Geometry: see drawing. Coordinates: mm, zero at the bounding-box minimum. A direction names the side the tool comes from. Round coordinates to 2 decimals unless told otherwise and drop trailing zeros. Write each loop counter-clockwise with the first axis right and the second up, starting at its lowest first coordinate (ties: lowest second). Pieces come first, ordered by that corner, then holes. Notation, with made-up numbers: M 38,16.25 L 64,16.25 A32 ccw 64,55.25 Z; hole C 63,2 d7. An arc over 180 degrees is marked long. Use a Markdown table: item, result.
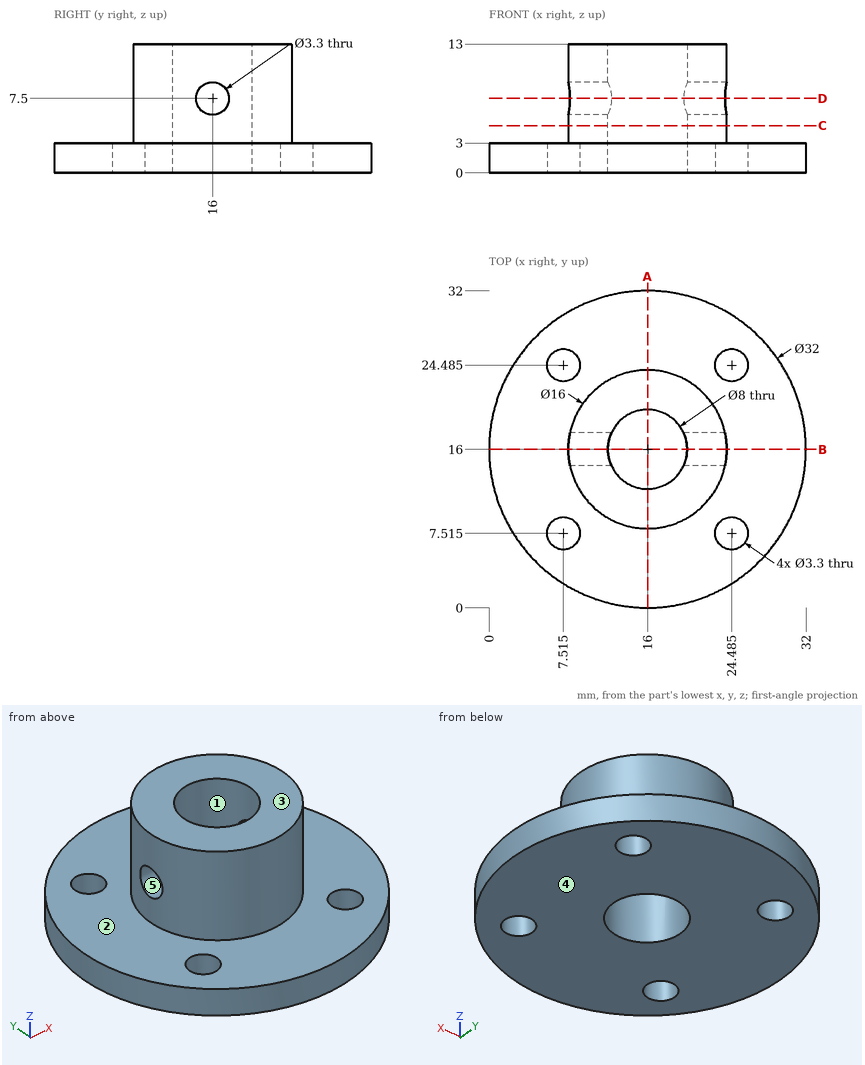
Q1. Mould query, pull axis Z, two halves, no side actions, for the marked faces 3, 4 and 5. Classes: +Z half, -Z half, draft (parallel to the pull), parting line (faces both ways), or undercut.
Results are:
| item | result |
|---|---|
| face 3 | +Z half |
| face 4 | -Z half |
| face 5 | undercut |
Q2. Section D-D on z = 7.5. Return loops of the section in (x, y), plus the area to 3 significant figures.
Results are:
| item | result |
|---|---|
| outline | M 8.17,14.35 A8 ccw 23.83,14.35 L 19.64,14.35 A4 cw 12.36,14.35 Z; M 8.17,17.65 L 12.36,17.65 A4 cw 19.64,17.65 L 23.83,17.65 A8 ccw Z |
| area | 124 mm^2 |
Q3. Section B-B on y = 16. Return loops of the section in (x, z), plus the area to 3 significant figures.
Results are:
| item | result |
|---|---|
| outline | M 0,0 L 12,0 L 12,5.85 L 8,5.85 L 8,3 L 0,3 Z; M 8,9.15 L 12,9.15 L 12,13 L 8,13 Z; M 20,0 L 32,0 L 32,3 L 24,3 L 24,5.85 L 20,5.85 Z; M 20,9.15 L 24,9.15 L 24,13 L 20,13 Z |
| area | 126 mm^2 |
Q4. First-contact query: pin 1 Ø5 at (x, y) = (9, 6.5) entering from +Z; pin 2 Ø4 at (y, z) = (16, 7.5) entering from -X; pin 3 Ø5 at (x, z) = (11.5, 9.5) entering from -Y. Flat tips, straight axial feed; report the tip coordinate or a pass-through.
Results are:
| item | result |
|---|---|
| pin 1 | z = 3 |
| pin 2 | x = 8 |
| pin 3 | y = 8.25 |
Q5. Section C-C on z = 4.75. Return loops of the section in (x, y), plus the area to 3 significant figures.
Results are:
| item | result |
|---|---|
| outline | C 16,16 d16; hole C 16,16 d8 |
| area | 151 mm^2 |
Q6. Section A-A on x = 16. Return loops of the section in (y, z), plus the area to 3 significant figures.
Results are:
| item | result |
|---|---|
| outline | M 0,0 L 12,0 L 12,13 L 8,13 L 8,3 L 0,3 Z; M 20,0 L 32,0 L 32,3 L 24,3 L 24,13 L 20,13 Z |
| area | 152 mm^2 |
Q7. Reachability of the marked faces 1 and 2 from +Z, -Z, +X, -X, +Y, -Y: full face, straight path, thin tool, end or side. Return the list, or none.
Results are:
| item | result |
|---|---|
| face 1 | +Z, -Z |
| face 2 | +Z |
Q8. Line query: L1, parallel to Z at x = 22.4, y = 16; L2, parallel to Z at x = 26.5, y = 22.5; L3, parallel to X at y = 14, z = 5 (1 decimal). Output: solid intervals per line, ascending.
Results are:
| item | result |
|---|---|
| L1 | 0 to 5.85, 9.15 to 13 |
| L2 | 0 to 3 |
| L3 | 8.3 to 12.5, 19.5 to 23.7 |
